Verification items for the finished model (mm, model axes). Face numbers are marked on the shaded views. Coordinates: 2 decimals unless noted, no trailing zeros. Order: outer loops, then holes, each group sorted by start corner. A loop starts at its lowest first (then second) coordinate and runs counter-clockwise, first axis right, second up. Notation, with made-up numbers: (-19, 49) -> (1, 49) arc R20 ccw to (1, 81) -> close; hole circle Ø6 at (76.25, 15). An arc over 180 degrees is marked (long way). Use CSV: the item, a comma, the result in double quotes. Start each with the question number.
1) Scan lines: line 1 along Y through (x, z) = (5, 2.3); line 2 along X through (y, z) = (3.5, 3.2); line 3 along X through (y, z) = (5, 4.4). Record each from-to range of solid material in increasing order.
2) Go/stop test with a flat-tipped pin: pin 1 (4 mm diameter, centred on x = 4, y = 7, fed in from -Z). Record where the tip stops, or that it passes through.
3) Sectioned sample at A-A on y = 4. Record the boundary of the cut face in (x, z), then the cut area to 3 significant figures.
4) Sectioned sample at B-B on x = 5. Record the boundary of the cut face in (y, z), then the cut area to 3 significant figures.
5) Sectioned sample at D-D on x = 9. Record the boundary of the cut face in (y, z), then the cut area to 3 significant figures.
6) Release check for a two-part mould opening along X. For the marked faces 1, 2 and 3 record: released by +X, released by -X, zero draft, split by the parting line, or undercut.
7) Sectioned sample at C-C on z = 0.7. Record the boundary of the cut face in (x, y), then the cut area to 3 significant figures.
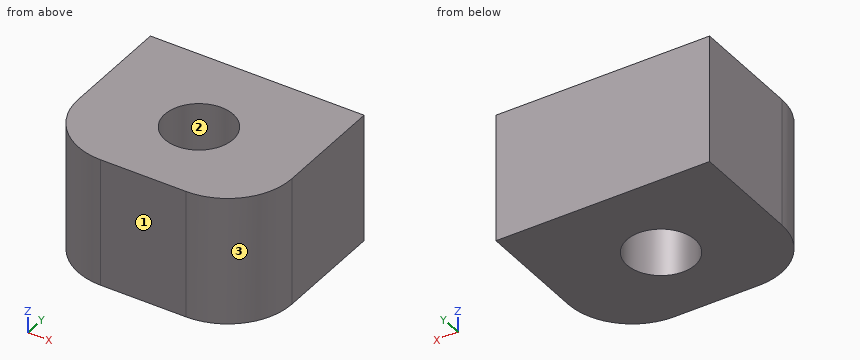
from build123d import *

# Parameters (mm, degrees)
CYLINDER_R     = 1.6
CYLINDER_DEPTH = 6
BOX_W          = 10
BOX_H          = 8.2
BOX_DEPTH      = 6
FILLET_R       = 3


with BuildPart() as obj1:
    # Cylinder → Cylinder (new body)
    with BuildSketch(Plane(origin=(5, 4, 0), x_dir=(1, 0, 0), z_dir=(0, 0, 1))):
        Circle(CYLINDER_R)
    extrude(amount=CYLINDER_DEPTH)


with BuildPart() as clampfillet:
    # Box → Box (new body)
    with BuildSketch(Plane.XY):
        with Locations((5, 4.1)):
            Rectangle(BOX_W, BOX_H)
    extrude(amount=BOX_DEPTH)

    # Cut: cut obj1
    add(obj1.part, mode=Mode.SUBTRACT)

    # Fillet
    fillet_edges = [clampfillet.edges().sort_by_distance(p)[0] for p in [
        (0, 0, 3),
        (10, 0, 3),
    ]]
    fillet(fillet_edges, radius=FILLET_R)


solid = clampfillet.part
Answers follow:
1,line 1,"y = 0 to 2.4, 5.6 to 8.2"
1,line 2,"x = 0 to 3.48, 6.52 to 10"
1,line 3,"x = 0 to 3.75, 6.25 to 10"
2,pin 1,"stops at z = 0"
3,outline,"(0, 0) -> (3.4, 0) -> (3.4, 6) -> (0, 6) -> close; (6.6, 0) -> (10, 0) -> (10, 6) -> (6.6, 6) -> close"
3,area,"40.8 mm²"
4,outline,"(0, 0) -> (2.4, 0) -> (2.4, 6) -> (0, 6) -> close; (5.6, 0) -> (8.2, 0) -> (8.2, 6) -> (5.6, 6) -> close"
4,area,"30.0 mm²"
5,outline,"(0.76, 0) -> (8.2, 0) -> (8.2, 6) -> (0.76, 6) -> close"
5,area,"44.6 mm²"
6,face 1,"zero draft"
6,face 2,"undercut"
6,face 3,"released by +X"
7,outline,"(0, 3) arc R3 ccw to (3, 0) -> (7, 0) arc R3 ccw to (10, 3) -> (10, 8.2) -> (0, 8.2) -> close; hole circle Ø3.2 at (5, 4)"
7,area,"70.1 mm²"
